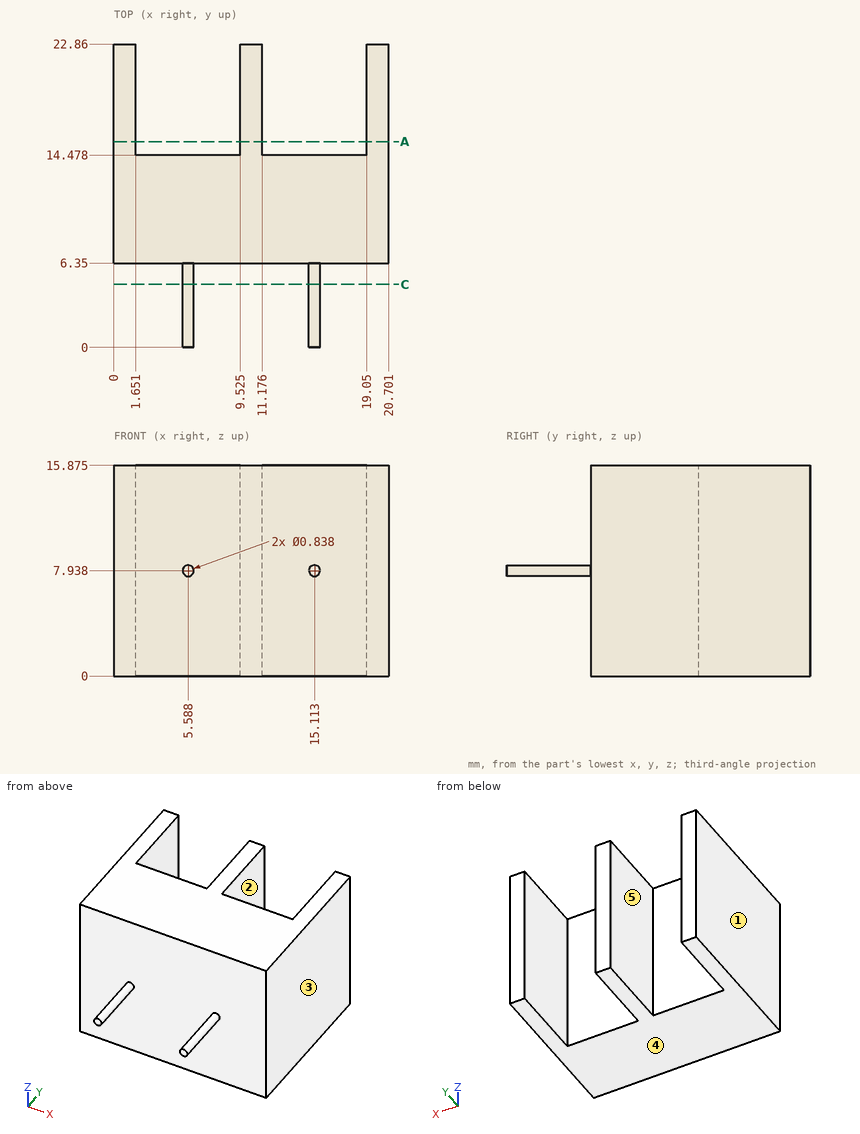
Geometry: see drawing. Coordinates: mm, zero at the bounding-box minimum. A direction names the side the tool comes from. Give positions to 0.01 mm unless a question says otherwise; leave off trailing zeros. Loops run counter-clockwise (first coordinate to the right, second up) from the corner with the lowest first, then second, coordinate; pieces in that order, holes last. Notation, with made-up numbers: (63, 86) - (71, 86) arc R21 ccw to (71, 118) - close; hole circle Ø4 at (52.25, 6.5). An arc over 180 degrees is marked (long way). Answer as CSV lines item,"result". Start each with the question number.
1. Pin query (flat end, axial travel): P1, Ø2.5, axis at x = 17, z = 5.5, coming from the +Y side; P2, Ø8, axis at x = 17.5, z = 13.5, coming from the -Y side. Return the tip coordinate at first contact, or that it passes through.
2. Draft query along X for the marked faces 3, 4 and 5. Return one class per face: released by +X, released by -X, zero draft, split by the parting line, or undercut.
3. Section C-C, the plane y = 4.75. Return loops of the section in (x, z).
4. Reachability of the marked faces 1 and 2 from +Z, -Z, +X, -X, +Y, -Y: full face, straight path, thin tool, end or side. Return the list, or none.
5. Section A-A, the plane y = 15.5. Give the number of separate pieces and of enclosed holes in the cut face.
6. Ray query, L1, parallel to Y at x = 13.5, z = 6.25; L2, parallel to Y at x = 10.25, z = 8.25; L3, parallel to Z at x = 5.5, y = 6. Return the intervals inside material, ascending.
Answers:
1,P1,"stops at y = 14.48"
1,P2,"stops at y = 6.35"
2,face 3,"released by +X"
2,face 4,"zero draft"
2,face 5,"undercut"
3,outline,"circle Ø0.84 at (5.59, 7.94); circle Ø0.84 at (15.11, 7.94)"
4,face 1,"+Z, -Z, -X, +Y, -Y"
4,face 2,"+Z, -Z, +Y"
5,separate pieces,"3"
5,enclosed holes,"0"
6,L1,"y = 6.35 to 14.48"
6,L2,"y = 6.35 to 22.86"
6,L3,"z = 7.53 to 8.35"
